Part model, mm, in its own coordinate system. Face numbers are marked on the shaded views. Coordinates: 2 decimals unless noted, no trailing zeros. Loops run counter-clockwise (first coordinate to the right, second up) from the corner with the lowest first, then second, coordinate; pieces in that order, holes last. Notation, with made-up numbers: M 51,34 L 105,34 A26 cw 105,69 Z; hole C 14,52.25 d4. An arc over 180 degrees is marked long. Answer as a JSON object with one key per item and string values. Group by question number.
1. Saw through at B-B on y = 111. Write the cut outline in (x, z), then the cut area to 3 significant figures.
2. Saw through at C-C on x = 33. Write the cut outline in (y, z).
3. Saw through at A-A on x = 49. Write the cut outline in (y, z).
4. Saw through at D-D on y = 53.5. Write the cut outline in (x, z), then the cut area to 3 significant figures.
5. Mould opens along X. For the marked faces 1, 2 and 3 say: released by +X, released by -X, zero draft, split by the parting line, or undercut.
6. Drill centre lines: L1, parallel to X at y = 25, z = 0; L2, parallel to Y at x = 16.5, z = 28.5; L3, parallel to Y at x = 22, z = 14. Where is each one in solid material? Low to high.
7. Drop flat-ended pins along their axis: pin 1 Ø1.5 at (x, z) = (55, 9) entering from +Y; pin 2 Ø5.5 at (x, z) = (11.7, -14.91) entering from -Y; pin 3 Ø1 at (y, z) = (56.5, -19.5) entering from +X; pin 4 Ø8 at (x, y) = (32, 22) entering from -Z. Give the stop position or say it passes through.
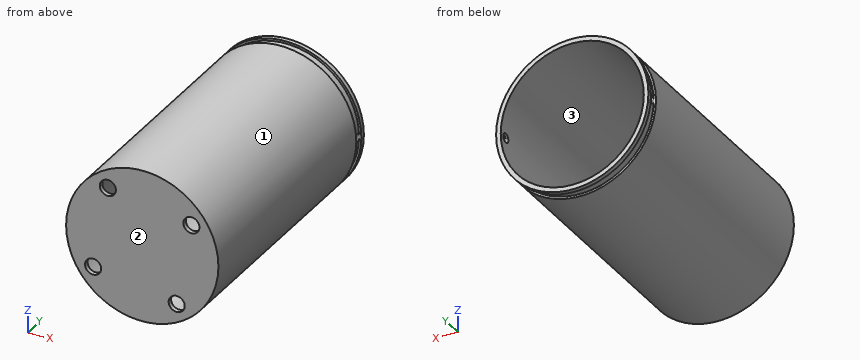
from build123d import *

# Parameters (mm, degrees)
ESQUISSE3_R             = 31
ENL_V_MAT_EXTRU_2_DEPTH = 113
ESQUISSE4_R             = 2
ENL_V_MAT_EXTRU_3_DEPTH = 64
ESQUISSE6_R             = 3.5
ENL_V_MAT_EXTRU_5_DEPTH = 10


with BuildPart() as part:
    # Esquisse1 → Révolution1 (revolve)
    with BuildSketch(Plane.XY):
        Polygon((0, 0), (0, 109), (1, 109), (1, 113), (0, 113), (0, 115), (33, 115), (33, 0), align=None)
    revolve(axis=Axis((33, 183.335721317, 0), (0, -1, 0)))

    # Esquisse3 → Enlèv. mat.-Extru.2 (cut)
    with BuildSketch(Plane(origin=(0, 115, 0), x_dir=(1, 0, 0), z_dir=(0, 1, 0))):
        with Locations(Location((33, 0, 0), (0, 0, 180))):
            Circle(ESQUISSE3_R)
    extrude(amount=-ENL_V_MAT_EXTRU_2_DEPTH, mode=Mode.SUBTRACT)

    # Esquisse4 → Enlèv. mat.-Extru.3 (cut)
    with BuildSketch(Plane(origin=(65, 0, 0), x_dir=(0, 0, -1), z_dir=(1, 0, 0))):
        with Locations(Location((0, 111, 0), (0, 0, 90))):
            Circle(ESQUISSE4_R)
    extrude(amount=-ENL_V_MAT_EXTRU_3_DEPTH, mode=Mode.SUBTRACT)

    # Esquisse6 → Enlèv. mat.-Extru.5 (cut)
    with BuildSketch(Plane.XZ):
        with Locations((54.297953152, 14.912987345)):
            Circle(ESQUISSE6_R)
        with Locations((18.087012655, 21.297953152)):
            Circle(ESQUISSE6_R)
        with Locations(Location((11.702046848, -14.912987345, 0), (0, 0, 180))):
            Circle(ESQUISSE6_R)
        with Locations(Location((47.912987345, -21.297953152, 0), (0, 0, 180))):
            Circle(ESQUISSE6_R)
    extrude(amount=-ENL_V_MAT_EXTRU_5_DEPTH, mode=Mode.SUBTRACT)


solid = part.part
Outcome:
{
 "1": {"outline": "M 1.06,-2 A32 ccw 64.94,-2 L 63.94,-2 A31 cw 2.06,-2 Z; M 1.06,2 L 2.06,2 A31 cw 63.94,2 L 64.94,2 A32 ccw Z", "area": "190 mm²"},
 "2": {"outline": "M 0,-33 L 109,-33 L 109,-32 L 113,-32 L 113,-33 L 115,-33 L 115,-31 L 2,-31 L 2,31 L 115,31 L 115,33 L 113,33 L 113,32 L 109,32 L 109,33 L 0,33 Z"},
 "3": {"outline": "M 0,-28.86 L 109,-28.86 L 109,-27.71 L 113,-27.71 L 113,-28.86 L 115,-28.86 L 115,-26.55 L 2,-26.55 L 2,-24.62 L 0,-24.62 Z; M 0,-17.97 L 2,-17.97 L 2,26.55 L 115,26.55 L 115,28.86 L 113,28.86 L 113,27.71 L 109,27.71 L 109,28.86 L 0,28.86 Z"},
 "4": {"outline": "C 33,0 d66; hole C 33,0 d62", "area": "402 mm²"},
 "5": {"face 1": "split by the parting line", "face 2": "zero draft", "face 3": "undercut"},
 "6": {"L1": "x = 0 to 2, 64 to 66", "L2": "y = 0 to 109, 113 to 115", "L3": "y = 0 to 2"},
 "7": {"pin 1": "stops at y = 2", "pin 2": "passes through", "pin 3": "stops at x = 59.98", "pin 4": "stops at z = -33"}
}
